```python
from build123d import *

# Parameters (mm, degrees)
SKETCH1_R           = 2.75
BOSS_EXTRUDE6_DEPTH = 3


with BuildPart() as part:
    # Sketch1 → Boss-Extrude6 (new body)
    with BuildSketch(Plane(origin=(0, 0, 0), x_dir=(1, 0, 0), z_dir=(0, 1, 0))):
        with BuildLine():
            Line((-45, -12.5), (45, -12.5))
            add(Edge.make_bspline(
                [(49.941104818, 8.442089367), (50.270924983, 7.993844293), (51.917772, 5.447061543), (54.055554594, -2.684937186), (49.028319605, -9.822821411), (45, -12.5)],
                knots=[0.210171728, 0.210171728, 0.210171728, 0.210171728, 0.264235121, 0.503984815, 1, 1, 1, 1], degree=3))
            Line((49.941104818, 8.442089367), (-37.395508702, 8.442089367))
            Line((-37.395508702, 8.442089367), (-37.395508702, 35.5))
            Line((-37.395508702, 35.5), (-55.5, 35.5))
            ThreePointArc((-55.5, 35.5), (-56.914213562, 34.914213562), (-57.5, 33.5))
            Line((-57.5, 33.5), (-57.5, 0))
            ThreePointArc((-57.5, 0), (-53.838834765, -8.838834765), (-45, -12.5))
        make_face()
        with Locations((45, 0)):
            Circle(SKETCH1_R, mode=Mode.SUBTRACT)
    extrude(amount=BOSS_EXTRUDE6_DEPTH)


solid = part.part
```
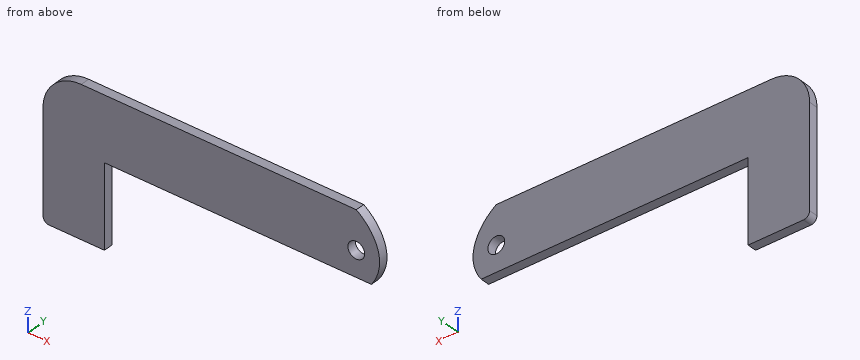
Geometry check sheet. Reference: the model listing, model coordinates, mm. Round coordinates to 2 decimals unless told otherwise and drop trailing zeros. Write each loop counter-clockwise with the first axis right and the second up, starting at its lowest first coordinate (ties: lowest second). Pieces come first, ordered by that corner, then holes. Notation, with made-up numbers: (-13, -21) -> (2, -21) arc R25 cw to (2, -3) -> close; hole circle Ø8 at (41, 45). An arc over 180 degrees is marked (long way). Put each result on its own line as item: value.
1) Cross-section at C-C, the plane x = 8.5. Enter the section's corners in (y, z).
Recorded:
outline: (0, -8.44) -> (3, -8.44) -> (3, 12.5) -> (0, 12.5) -> close
2) Cross-section at B-B, the plane z = -17.5. Enter the section's corners in (x, y), plus the area to 3 significant figures.
Recorded:
outline: (-57.5, 0) -> (-37.4, 0) -> (-37.4, 3) -> (-57.5, 3) -> close
area: 60.3 mm2
3) Thickness scan on probe 1 along X at (y, z) = (0.95, 0); probe 2 along Z at (x, y) = (45, 2.15); probe 3 along X at (y, z) = (2.7, -31). Record the ranges inside material, lowest first. Write a range as from..to.
Recorded:
probe 1: x = -57.5..42.25, 47.75..52.62
probe 2: z = -8.44..-2.75, 2.75..12.5
probe 3: x = -57.5..-37.4
4) Depth check by flat-ended pin: P1, Ø3.5, axis at x = 45, z = 0, coming from the -Y side. Enter the tip coordinate at first touch or a pass-through.
Recorded:
P1: passes through
5) Cross-section at A-A, the plane x = 43.5. Enter the section's corners in (y, z), plus the area to 3 significant figures.
Recorded:
outline: (0, -8.44) -> (3, -8.44) -> (3, -2.3) -> (0, -2.3) -> close; (0, 2.3) -> (3, 2.3) -> (3, 12.5) -> (0, 12.5) -> close
area: 49.0 mm2
